Build history of the part. All positions in model axes, mm. Face numbers are marked on the shaded views. Round coordinates to 2 decimals unless told otherwise and drop trailing zeros. Write each loop counter-clockwise with the first axis right and the second up, starting at its lowest first coordinate (ties: lowest second). Pieces come first, ordered by that corner, then holes. Notation, with made-up numbers: (68, 70) - (122, 70) arc R25 ccw to (122, 104) - close; hole circle Ø1 at (-24.5, 57.5). An arc over 180 degrees is marked (long way). Write each question's results on one line, items separated by ' | '.
from build123d import *

# Parameters (mm, degrees)
F0_R     = 1.7145
F1_DEPTH = 1.778
F0_R_2   = 12.7
F2_DEPTH = 3.81
F3_R     = 1.524
F5_DEPTH = 81.789
F6_DEPTH = 81.789


with BuildPart() as f1:
    # F0 (on Front) → F1 (new body, symmetric)
    with BuildSketch(Plane.XZ):
        with BuildLine():
            Line((18.6069666262, -2.2111574336), (18.6069666262, -4.4971574336))
            Line((18.6069666262, -4.4971574336), (21.4009666262, -4.4971574336))
            Line((21.4009666262, -4.4971574336), (21.4009666262, -7.7991574336))
            Line((21.4009666262, -7.7991574336), (97.6009666262, -7.7991574336))
            ThreePointArc((97.6009666262, -7.7991574336), (100.3949666262, -5.0051574336), (97.6009666262, -2.2111574336))
            Line((97.6009666262, -2.2111574336), (18.6069666262, -2.2111574336))
        make_face()
        with Locations((31.9419666262, -4.7511574336)):
            Circle(F0_R, mode=Mode.SUBTRACT)
    extrude(amount=F1_DEPTH, both=True)

    # F0 (on Front) → F2 (join, symmetric)
    with BuildSketch(Plane.XZ):
        with BuildLine():
            ThreePointArc((-35.3680333738, -4.4971574336), (-34.9216641084, -5.5747881681), (-33.8440333738, -6.0211574336))
            Line((-33.8440333738, -6.0211574336), (17.0829666262, -6.0211574336))
            ThreePointArc((17.0829666262, -6.0211574336), (18.1605973607, -5.5747881681), (18.6069666262, -4.4971574336))
            Line((18.6069666262, -4.4971574336), (18.6069666262, -2.2111574336))
            Line((18.6069666262, -2.2111574336), (18.6069666262, -1.6228641659))
            ThreePointArc((18.6069666262, -1.6228641659), (18.2019597184, -0.5882480731), (17.2022022436, -0.1035357395))
            ThreePointArc((17.2022022436, -0.1035357395), (8.1933226976, 3.4532292373), (2.7294715366, 11.4505299235))
            ThreePointArc((2.7294715366, 11.4505299235), (-16.1638720044, 30.8082187838), (-35.3680333738, 11.7588425664))
            Line((-35.3680333738, 11.7588425664), (-35.3680333738, -4.4971574336))
        make_face()
        with Locations((-16.3180333738, 11.7588425664)):
            Circle(F0_R_2, mode=Mode.SUBTRACT)
    extrude(amount=F2_DEPTH, both=True)

    # F3
    f3_edges = [f1.edges().sort_by_distance(p)[0] for p in [
        (-16.163872, -3.81, 30.808219),
        (-16.163872, 3.81, 30.808219),
    ]]
    fillet(f3_edges, radius=F3_R)

    # F4 (on face) → F5 (cut, through all)
    with BuildSketch(Plane.YZ.offset(18.6069666262)):
        Polygon((-2.286, -2.2111574336), (-2.286, -3.0600107998), (2.6955511421, -2.2111574336), align=None)
    extrude(amount=F5_DEPTH, mode=Mode.SUBTRACT)

    # F4 (on face) → F6 (cut, through all)
    with BuildSketch(Plane.YZ.offset(18.6069666262)):
        Polygon((-2.286, -2.2111574336), (-2.286, -3.0600107998), (2.6955511421, -2.2111574336), align=None)
    extrude(amount=F6_DEPTH, mode=Mode.SUBTRACT)


solid = f1.part
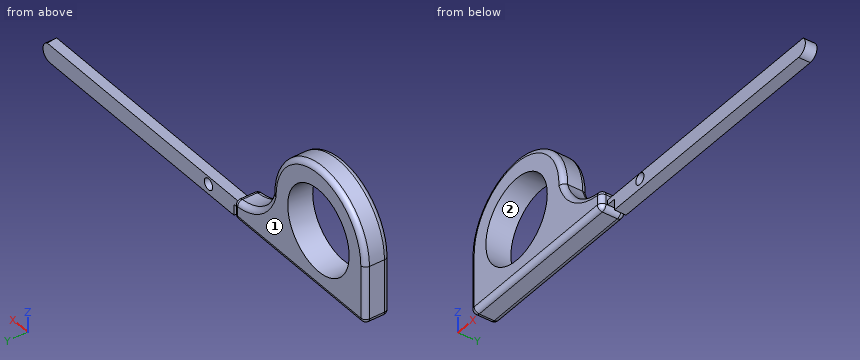
(1) Drill centre lines: probe 1 along X at (y, z) = (-2, 12); probe 2 along X at (y, z) = (0, -5); probe 3 along Z at (x, y) = (-21, 0). Where is each one in solid material? Low to high. Write a range as [from, to].
Worked answers:
probe 1: x = [-35.37, -29.02], [-3.62, 2.73] | probe 2: x = [-35.28, 18.52], [21.4, 30.25], [33.64, 100.39] | probe 3: z = [-6.02, -0.05], [23.56, 30.22]
(2) Flat gauge pins, fed straight in: pin 1 Ø3.5 at (x, y) = (-14, -0.5) entering from -Z; pin 2 Ø4 at (x, z) = (73.5, -6) entering from -Y; pin 3 Ø5.5 at (x, z) = (31.94, -4.75) entering from +Y; pin 4 Ø20.5 at (x, z) = (-16.32, 11.76) entering from -Y. Where does each tip first touch, or does it go through?
Worked answers:
pin 1: stops at z = -6.02 | pin 2: stops at y = -1.78 | pin 3: stops at y = 1.78 | pin 4: passes through
(3) Slice it at A-A, the plane y = -0.5. Write the cut outline in (x, z), and give its area (3 significant figures).
Worked answers:
outline: (-35.37, -4.5) arc R1.52 ccw to (-33.84, -6.02) - (17.08, -6.02) arc R1.52 ccw to (18.61, -4.5) - (21.4, -4.5) - (21.4, -7.8) - (97.6, -7.8) arc R2.79 ccw to (99.26, -2.76) - (18.61, -2.76) - (18.61, -1.62) arc R1.52 ccw to (17.2, -0.1) arc R16.51 cw to (2.73, 11.45) arc R19.05 ccw (long way) to (-35.37, 11.76) - close; hole circle Ø25.4 at (-16.32, 11.76); hole circle Ø3.43 at (31.94, -4.75) | area: 1,270 mm2
(4) Slice it at B-B, the plane x = 76. Write the cut outline in (y, z), and give its area (3 significant figures).
Worked answers:
outline: (-1.78, -7.8) - (1.78, -7.8) - (1.78, -2.37) - (-1.78, -2.97) - close | area: 18.2 mm2
(5) Two-plate mould, pull along Z, no slides. Class the marked faces 1 and 2: released by +Z, released by -Z, zero draft, split by the parting line, or undercut.
Worked answers:
face 1: zero draft | face 2: undercut
